```python
from build123d import *

# Parameters (mm, degrees)
SKETCH_2_R          = 1.5
CUT_EXTRUDE_1_DEPTH = 31.356218473
CUT_EXTRUDE_START   = 4
SKETCH_3_R          = 3.25
CUT_EXTRUDE_2_DEPTH = 2
EXTRUDE_START       = 6
EXTRUDE_1_DEPTH     = 6
SKETCH_5_R          = 7.5
CUT_EXTRUDE_3_DEPTH = 1
CHAMFER_1_SIZE      = 0.5
CHAMFER_2_SIZE      = 0.5
CUT_EXTRUDE_4_DEPTH = 6
EXTRUDE_2_DEPTH     = 6


with BuildPart() as part:
    # 草图1 → 旋转1 (revolve)
    with BuildSketch(Plane.XY):
        Polygon((-4.5, 0), (-20.5, 0), (-20.5, 4), (-7, 4), (-7, 6.2), (-6.45, 6.2), (-6.45, 7.6), (-7, 7.6), (-7, 9), (-4.5, 9), align=None)
    revolve(axis=Axis((0, 7, 0), (0, -1, 0)))

    # 草图2 → 切除-拉伸1 (cut, through all)
    with BuildSketch(Plane(origin=(0, 0, 0), x_dir=(1, 0, 0), z_dir=(0, 1, 0))):
        with Locations(Location((-16, 0, 0), (0, 0, 180))):
            Circle(SKETCH_2_R)
        with Locations(Location((0, 16, 0), (0, 0, 180))):
            Circle(SKETCH_2_R)
        with Locations(Location((16, 0, 0), (0, 0, 180))):
            Circle(SKETCH_2_R)
    extrude(amount=CUT_EXTRUDE_1_DEPTH, mode=Mode.SUBTRACT)

    # 草图3 → 切除-拉伸2 (cut)
    with BuildSketch(Plane(origin=(0, 0, 0), x_dir=(1, 0, 0), z_dir=(0, 1, 0)).offset(CUT_EXTRUDE_START)):
        with Locations(Location((-16, 0, 0), (0, 0, 180))):
            Circle(SKETCH_3_R)
        with Locations(Location((0, 16, 0), (0, 0, 180))):
            Circle(SKETCH_3_R)
        with Locations(Location((16, 0, 0), (0, 0, 180))):
            Circle(SKETCH_3_R)
    extrude(amount=-CUT_EXTRUDE_2_DEPTH, mode=Mode.SUBTRACT)

    # 草图4 → 凸台-拉伸1 (add)
    with BuildSketch(Plane(origin=(0, 4, 0), x_dir=(1, 0, 0), z_dir=(0, 1, 0)).offset(EXTRUDE_START)):
        with BuildLine():
            Line((7.5, -12), (-7.5, -12))
            Line((-7.5, -12), (-7.5, -19.078784028))
            ThreePointArc((-7.5, -19.078784028), (0, -20.5), (7.5, -19.078784028))
            Line((7.5, -19.078784028), (7.5, -12))
        make_face()
    extrude(amount=-EXTRUDE_1_DEPTH)

    # 草图5 → 切除-拉伸3 (cut)
    with BuildSketch(Plane.XZ):
        Circle(SKETCH_5_R)
    extrude(amount=-CUT_EXTRUDE_3_DEPTH, mode=Mode.SUBTRACT)

    # 倒角1
    chamfer_1_edges = [part.edges().sort_by_distance(p)[0] for p in [
        (4.5, 1, 0),
        (4.5, 9, 0),
    ]]
    chamfer(chamfer_1_edges, length=CHAMFER_1_SIZE)

    # 倒角2
    chamfer_2_edges = [part.edges().sort_by_distance(p)[0] for p in [
        (7, 9, 0),
    ]]
    chamfer(chamfer_2_edges, length=CHAMFER_2_SIZE)

    # 草图6 → 切除-拉伸4 (cut)
    with BuildSketch(Plane(origin=(0, 10, 0), x_dir=(1, 0, 0), z_dir=(0, 1, 0))):
        Polygon((1.967727288, -14.033683215), (-1.353682174, -21.493691009), (7.5, -20.908921831), (7.5, -12), (-2.6, -12), align=None)
    extrude(amount=-CUT_EXTRUDE_4_DEPTH, mode=Mode.SUBTRACT)

    # 草图7 → 凸台-拉伸2 (add)
    with BuildSketch(Plane(origin=(0, 4, 0), x_dir=(1, 0, 0), z_dir=(0, 1, 0)).offset(EXTRUDE_START)):
        with BuildLine():
            Line((-2.6, -12), (3.073111454, -13.953408927))
            Line((3.073111454, -13.953408927), (0.824652926, -20.483406639))
            ThreePointArc((0.824652926, -20.483406639), (-0.038915526, -20.499963063), (-0.902414897, -20.480128109))
            Line((-0.902414897, -20.480128109), (1.967727288, -14.033683215))
            Line((1.967727288, -14.033683215), (-2.6, -12))
        make_face()
    extrude(amount=-EXTRUDE_2_DEPTH)


solid = part.part
```
Design review of the part built by this model. Coordinates are the model's own, in mm. A direction names the side the tool comes from. Coordinates: 2 decimals unless noted, no trailing zeros. Loops run counter-clockwise (first coordinate to the right, second up) from the corner with the lowest first, then second, coordinate; pieces in that order, holes last. Notation, with made-up numbers: M -15,14.25 L 23,14.25 A26 ccw 23,33.25 Z; hole C -39,23.5 d4. An arc over 180 degrees is marked long. One line per question, with ' | ' between items.
(1) We need section A-A (y = 2.5). Give the boundary of the cut face in (x, z), and give its area (3 significant figures).
Filled in:
outline: C 0,0 d41; hole C -16,0 d6.5; hole C 0,0 d9; hole C 0,-16 d6.5; hole C 16,0 d6.5 | area: 1,160 mm^2
(2) We need section C-C (z = -16). Give the boundary of the cut face in (x, y), and give its area (3 significant figures).
Filled in:
outline: M -12.82,0 L -1.5,0 L -1.5,2 L -3.25,2 L -3.25,4 L -12.82,4 Z; M 1.5,0 L 12.82,0 L 12.82,4 L 3.25,4 L 3.25,2 L 1.5,2 Z | area: 83.5 mm^2
(3) Draft analysis for pull direction Y (two halves, no side actions). For faces 1 (the face through (-6.466, 8.056, 2.681)), 2 (the face through (-3, 6.2, 6)), 3 (the face through (9, 0, 0)), state which applies: released by +Y, released by -Y, zero draft, split by the parting line, or undercut.
Filled in:
face 1: zero draft | face 2: undercut | face 3: released by -Y
(4) We need section B-B (x = -16). Give the boundary of the cut face in (y, z).
Filled in:
outline: M 0,-12.82 L 4,-12.82 L 4,-3.25 L 2,-3.25 L 2,-1.5 L 0,-1.5 Z; M 0,1.5 L 2,1.5 L 2,3.25 L 4,3.25 L 4,12.82 L 0,12.82 Z
(5) We need section D-D (z = 0). Count the separate pieces of the cut face and the enclosed holes in it, and give its area (3 significant figures).
Filled in:
separate pieces: 4 | enclosed holes: 0 | area: 107 mm^2
(6) For pin 1 Ø12 at (x, z) = (0, 0) entering from +Y; pin 2 Ø7 at (x, z) = (-17.5, 0.5) entering from +Y; pin 3 Ø4.5 at (x, z) = (-0.5, -0.5) entering from -Y; pin 4 Ø2 at (x, z) = (1, -16.5) entering from +Y, all flat-tipped, find the tip position at first contact; note any pin that passes through.
Filled in:
pin 1: stops at y = 9 | pin 2: stops at y = 4 | pin 3: passes through | pin 4: stops at y = 2
(7) Machinability: for faces 4 (the face through (-6.466, 5.115, 2.681)), 5 (the face through (-2, 9, 5)), 6 (the face through (-7.493, 0.493, 0.33)), 7 (the face through (0.197, 7.042, 12.963)), which of the approach directions +Z, -Z, +X, -X, +Y, -Y give a long, thin tool a straight path to every point of the face, cutting with its end or side? Answer none if there is none.
Filled in:
face 4: +Y | face 5: -Z, +X, -X, +Y | face 6: -Y | face 7: +X, +Y
(8) Wall thickness on probe 1 along Z at (x, y) = (0, 3); probe 2 along Z at (x, y) = (-2, 4.5); probe 3 along X at (y, z) = (7.25, 0): over which ranges is each line inside the solid? List them lowest first.
Filled in:
probe 1: z = -20.5 to -19.25, -12.75 to -4.5, 4.5 to 20.5 | probe 2: z = -6.71 to -4.03, 4.03 to 6.71, 12.21 to 20.4 | probe 3: x = -6.45 to -4.5, 4.5 to 6.45
